```python
from build123d import *

# Parameters (mm, degrees)
F0_W     = 210
F0_H     = 297
F1_DEPTH = 8
F2_R     = 5.5
F3_DEPTH = 8.001
F4_R     = 56.75
F4_R_2   = 3.25
F5_DEPTH = 8.001
F6_R     = 5.125
F6_R_2   = 2.25
F7_DEPTH = 8.001


with BuildPart() as f1:
    # F0 (on Front) → F1 (new body)
    with BuildSketch(Plane.XZ):
        with Locations((105, 148.5)):
            Rectangle(F0_W, F0_H)
    extrude(amount=-F1_DEPTH)

    # F2 (on face) → F3 (cut, through all)
    with BuildSketch(Plane.XZ):
        with Locations((14, 122)):
            Circle(F2_R)
        with Locations((31.5, 63.5)):
            Circle(F2_R)
        with Locations((81, 82)):
            Circle(F2_R)
        with Locations((49, 13.5)):
            Circle(F2_R)
        with BuildLine():
            ThreePointArc((104.039609, 48), (93.77548, 50.834696), (86.42092, 58.535235))
            ThreePointArc((86.42092, 58.535235), (48.814136, 63.738258), (55.327996, 26.336236))
            ThreePointArc((55.327996, 26.336236), (61.152657, 21.058135), (63.311271, 13.5))
            Line((63.311271, 13.5), (63.311271, 0))
            Line((63.311271, 0), (210, 0))
            Line((210, 0), (210, 77.888055))
            Line((210, 77.888055), (185.96981, 53.857864))
            ThreePointArc((185.96981, 53.857864), (179.481343, 49.522409), (171.827674, 48))
            Line((171.827674, 48), (104.039609, 48))
        make_face()
    extrude(amount=-F3_DEPTH, mode=Mode.SUBTRACT)

    # F4 (on face) → F5 (cut, through all)
    with BuildSketch(Plane.XZ):
        with Locations((129, 205.934511)):
            Circle(F4_R)
        with Locations((95.75, 263.5252)):
            Circle(F4_R_2)
        with Locations((162.25, 263.5252)):
            Circle(F4_R_2)
        with Locations((95.75, 148.343821)):
            Circle(F4_R_2)
        with Locations((162.25, 148.343821)):
            Circle(F4_R_2)
    extrude(amount=-F5_DEPTH, mode=Mode.SUBTRACT)

    # F6 (on face) → F7 (cut, through all)
    with BuildSketch(Plane.XZ):
        with BuildLine():
            Line((177.889947, 111.799242), (128.649559, 120.48165))
            ThreePointArc((128.649559, 120.48165), (122.712473, 116.324458), (126.869665, 110.387371))
            Line((126.869665, 110.387371), (176.110053, 101.704962))
            ThreePointArc((176.110053, 101.704962), (182.04714, 105.862155), (177.889947, 111.799242))
        make_face()
        with Locations((36.723409, 162.174419)):
            Circle(F6_R)
        with Locations((45.894034, 212.34313)):
            Circle(F6_R_2)
    extrude(amount=-F7_DEPTH, mode=Mode.SUBTRACT)


solid = f1.part
```
Verification items for the finished model (mm, model axes). A direction names the side the tool comes from. Coordinates: 2 decimals unless noted, no trailing zeros. Order: outer loops, then holes, each group sorted by start corner. A loop starts at its lowest first (then second) coordinate and runs counter-clockwise, first axis right, second up. Notation, with made-up numbers: (5.25, -28.75) -> (19.25, -28.75) arc R26 ccw to (19.25, -1.75) -> close; hole circle Ø5 at (60.5, 76). An arc over 180 degrees is marked (long way). Put each result on its own line as item: value. Start each with the question number.
1) Go/stop test with a flat-tipped pin: pin 1 (2.5 mm diameter, centred on x = 126, y = 4.5, fed in from -Z). Record where the tip stops, or that it passes through.
2) Release check for a two-part mould opening along X. For faces 1 (the flat face through (104, 0, 151)), 2 (the cylindrical face through (61.093, 3.944, 21.153)), 3 (the cylindrical face through (155.19, 3.94, 155.59)) record: pulls with the +X half, pulls with the -X half, needs draft (parallel to the pull), parting line crosses it, or undercut.
3) Material ranges on L1, parallel to X at y = 6.75, z = 263; L2, parallel to Z at x = 31.5, y = 6.5; L3, parallel to Z at x = 156, y = 7.25, recorded low to high.
4) Cross-section at D-D (x = 162.25). Enter the section's corners in (y, z), plus the area to 3 significant figures.
5) Cross-section at B-B (z = 63.5). Enter the section's corners in (x, y), plus the area to 3 significant figures.
6) Cross-section at A-A (x = 81). Enter the section's corners in (y, z), plus the area to 3 significant figures.
7) Cross-section at C-C (y = 5.75). State how many separate pieces and enclosed holes the cut face has, plus the area to 3 significant figures.
8) Tool access check on faces 4 (the cylindrical face through (93.905, 3.944, 50.758)), 5 (the flat face through (63.311, 4, 7)), 6 (the flat face through (151.145, 3.944, 106.107)). Record the directions out of +Z, -Z, +X, -X, +Y, -Y that give a thin tool (end or side, any length) a straight path to the whole face; none if there is none.
Geometry check:
1. pin 1: stops at z = 48
2. face 1: needs draft
2. face 2: pulls with the +X half
2. face 3: undercut
3. L1: x = 0 to 92.54, 98.96 to 159.04, 165.46 to 210
3. L2: z = 0 to 58, 69 to 297
3. L3: z = 48 to 105.25, 115.66 to 156.02, 255.85 to 297
4. outline: (0, 48) -> (8, 48) -> (8, 104.15) -> (0, 104.15) -> close; (0, 114.56) -> (8, 114.56) -> (8, 145.09) -> (0, 145.09) -> close; (0, 151.59) -> (8, 151.59) -> (8, 159.95) -> (0, 159.95) -> close; (0, 251.92) -> (8, 251.92) -> (8, 260.28) -> (0, 260.28) -> close; (0, 266.78) -> (8, 266.78) -> (8, 297) -> (0, 297) -> close
4. area: 1,070 mm^2
5. outline: (0, 0) -> (26, 0) -> (26, 8) -> (0, 8) -> close; (37, 0) -> (48.59, 0) -> (48.59, 8) -> (37, 8) -> close; (82.85, 0) -> (195.61, 0) -> (195.61, 8) -> (82.85, 8) -> close
5. area: 1,200 mm^2
6. outline: (0, 65.27) -> (8, 65.27) -> (8, 76.5) -> (0, 76.5) -> close; (0, 87.5) -> (8, 87.5) -> (8, 175.66) -> (0, 175.66) -> close; (0, 236.21) -> (8, 236.21) -> (8, 297) -> (0, 297) -> close
6. area: 1,280 mm^2
7. separate pieces: 1
7. enclosed holes: 12
7. area: 42,300 mm^2
8. face 4: -Z, +Y, -Y
8. face 5: -Z, +X, +Y, -Y
8. face 6: +Y, -Y
